The figure shows three views and two pictorial views of one solid part (mm, origin at its lowest corner). Answer the questions. Coordinates: 2 decimals unless noted, no trailing zeros. Order: outer loops, then holes, each group sorted by start corner. A loop starts at its lowest first (then second) coordinate and runs counter-clockwise, first axis right, second up. Notation, with made-up numbers: (-36.75, -32) -> (12.25, -32) arc R6 cw to (12.25, -26) -> close; hole circle Ø4 at (70, -32.75). An arc over 180 degrees is marked (long way). Write item = value, one per line. Start each with the question number.
Q1. A flat-ended cylindrical pin translates along its axis: pin 1 (12 mm diameter, centred on x = 12.7, y = 228.6, fed in from +Z). Find the tip coordinate at first contact, or state that the pin passes through.
Q2. The part is cut by section A-A, the plane x = 12.7. Determine the outline of the cut face in (y, z).
Q3. Straight lines are drawn through the part: L1, parallel to Y at x = 12.7, z = 3.4; L2, parallel to X at y = 15.5, z = 3.4 (1 decimal). For each, find the intervals that lie inside material, in ascending order. Write a range as from..to.
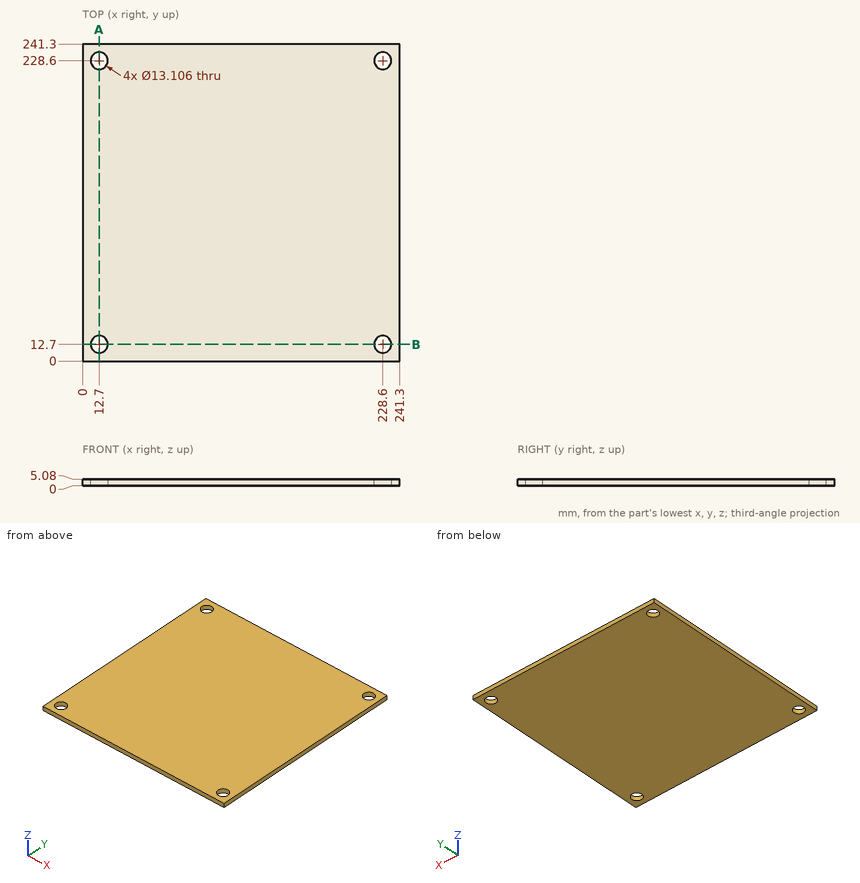
Model answer:
q1.pin_1 = through
q2.outline = (0, 0) -> (6.15, 0) -> (6.15, 5.08) -> (0, 5.08) -> close; (19.25, 0) -> (222.05, 0) -> (222.05, 5.08) -> (19.25, 5.08) -> close; (235.15, 0) -> (241.3, 0) -> (241.3, 5.08) -> (235.15, 5.08) -> close
q3.L1 = 0..6.15, 19.25..222.05, 235.15..241.3
q3.L2 = 0..6.8, 18.6..222.7, 234.5..241.3
